Could you check a few things on this drawing? It's one solid part, dimensions in mm from its lowest x, y, z. Give positions to 0.01 mm unless a question says otherwise; leave off trailing zeros. Loops run counter-clockwise (first coordinate to the right, second up) from the corner with the lowest first, then second, coordinate; pieces in that order, holes last.
1. Imagine slicing it at C-C (z = 125.5). List the corners of the cut face in (x, y) for me.
2. For P1, Ø2, axis at x = 57, y = 1, coming from the -Z side, with a flat end and sliding along its axis, tell me the tip position at first contact or that it passes through.
3. I need wall thicknesses on line 1 along Z through (x, y) = (10.5, 5.25); line 2 along X through (y, z) = (4, 55) (1 decimal); line 3 along X through (y, z) = (2.25, 49). Which ranges of each line are inside material? Lowest first, please.
4. Imagine slicing it at A-A (y = 4.25). List the corners of the cut face in (x, z) for me, plus the area to 3 significant figures.
5. Imagine slicing it at B-B (x = 14). Count the separate pieces of the cut face and the enclosed holes in it.
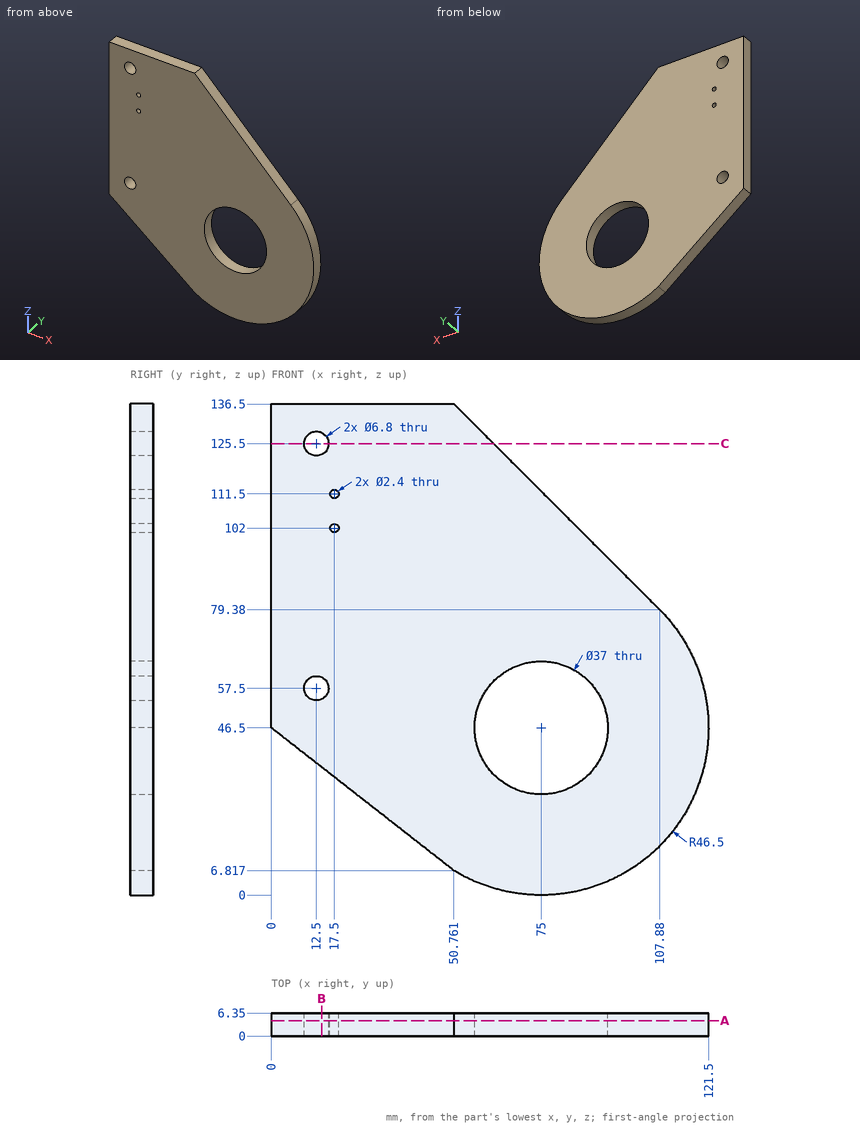
Derived:
1. outline: (0, 0) - (9.1, 0) - (9.1, 6.35) - (0, 6.35) - close; (15.9, 0) - (61.76, 0) - (61.76, 6.35) - (15.9, 6.35) - close
2. P1: stops at z = 3.22
3. line 1: z = 38.29 to 54.75, 60.25 to 122.75, 128.25 to 136.5
3. line 2: x = 0 to 10.2, 14.8 to 58.6, 91.4 to 120.7
3. line 3: x = 0 to 56.67, 93.33 to 121.43
4. outline: (0, 46.5) - (50.76, 6.82) arc R46.5 ccw to (107.88, 79.38) - (50.76, 136.5) - (0, 136.5) - close; hole circle Ø6.8 at (12.5, 57.5); hole circle Ø6.8 at (12.5, 125.5); hole circle Ø2.4 at (17.5, 102); hole circle Ø2.4 at (17.5, 111.5); hole circle Ø37 at (75, 46.5)
4. area: 11,000 mm2
5. separate pieces: 3
5. enclosed holes: 0
